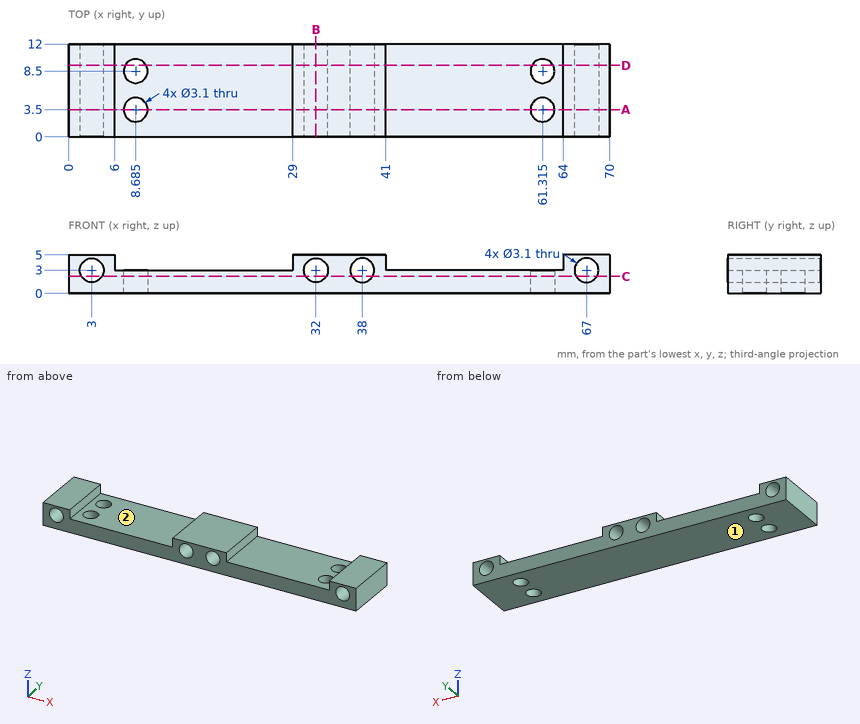
The figure shows three views and two pictorial views of one solid part (mm, origin at its lowest corner). Answer the questions. A direction names the side the tool comes from. Give positions to 0.01 mm unless a question says otherwise; leave off trailing zeros. Loops run counter-clockwise (first coordinate to the right, second up) from the corner with the lowest first, then second, coordinate; pieces in that order, holes last. Notation, with made-up numbers: (73, 51) - (111, 51) arc R17 ccw to (111, 58) - close; hole circle Ø10 at (88.5, 68.25). An arc over 180 degrees is marked (long way). Answer in a Markdown table with one row per item.
(1) Consider L1, parallel to Z at x = 38, y = 3.25; L2, parallel to Z at x = 13.5, y = 9; L3, parallel to Z at x = 66, y = 11. Determine where each line is inside the solid, lowest interval first. Write a range as [from, to].
Results list:
| item | result |
|---|---|
| L1 | z = [0, 1.45], [4.55, 5] |
| L2 | z = [0, 3] |
| L3 | z = [0, 1.82], [4.18, 5] |
(2) Section D-D (y = 9.25) is taken. Give the vertices of the cut face in (x, z).
Results list:
| item | result |
|---|---|
| outline | (0, 0) - (7.33, 0) - (7.33, 3) - (6, 3) - (6, 5) - (0, 5) - close; (10.04, 0) - (59.96, 0) - (59.96, 3) - (41, 3) - (41, 5) - (29, 5) - (29, 3) - (10.04, 3) - close; (62.67, 0) - (70, 0) - (70, 5) - (64, 5) - (64, 3) - (62.67, 3) - close; hole circle Ø3.1 at (3, 3); hole circle Ø3.1 at (32, 3); hole circle Ø3.1 at (38, 3); hole circle Ø3.1 at (67, 3) |
(3) Section B-B (x = 32) is taken. Give the vertices of the cut face in (y, z).
Results list:
| item | result |
|---|---|
| outline | (0, 0) - (12, 0) - (12, 1.45) - (0, 1.45) - close; (0, 4.55) - (12, 4.55) - (12, 5) - (0, 5) - close |
(4) Section A-A (y = 3.5) is taken. Give the vertices of the cut face in (x, z) (3 decimals).
Results list:
| item | result |
|---|---|
| outline | (0, 0) - (7.135, 0) - (7.135, 3) - (6, 3) - (6, 5) - (0, 5) - close; (10.235, 0) - (59.765, 0) - (59.765, 3) - (41, 3) - (41, 5) - (29, 5) - (29, 3) - (10.235, 3) - close; (62.865, 0) - (70, 0) - (70, 5) - (64, 5) - (64, 3) - (62.865, 3) - close; hole circle Ø3.1 at (3, 3); hole circle Ø3.1 at (32, 3); hole circle Ø3.1 at (38, 3); hole circle Ø3.1 at (67, 3) |
(5) A flat-ended cylindrical pin translates along its axis: pin 1 Ø2 at (x, y) = (21, 7) entering from +Z. Find the tip coordinate at first contact, or state that the pin passes through.
Results list:
| item | result |
|---|---|
| pin 1 | stops at z = 3 |
(6) A tool of negligible diameter and unlimited length cuts with its end or side. For the marked faces 1 and 2, from which of +Z, -Z, +X, -X, +Y, -Y can it reach the whole face along a straight path? Write none if from no direction.
Results list:
| item | result |
|---|---|
| face 1 | -Z, +X, -X, +Y, -Y |
| face 2 | +Z, +Y, -Y |
(7) Section C-C (z = 2.2) is taken. State how many separate pieces and enclosed holes the cut face has, and give its area (3 significant figures).
Results list:
| item | result |
|---|---|
| separate pieces | 5 |
| enclosed holes | 4 |
| area | 682 mm² |
